```python
from build123d import *

# Parameters (mm, degrees)
F0_W     = 65
F0_H     = 83
F0_R     = 2.75
F1_DEPTH = 5
F2_SIZE  = 10


with BuildPart() as f1:
    # F0 (on Front) → F1 (new body)
    with BuildSketch(Plane.XZ):
        with Locations((32.5, 41.5)):
            Rectangle(F0_W, F0_H)
        with Locations((17, 14)):
            Circle(F0_R, mode=Mode.SUBTRACT)
        with Locations((47, 14)):
            Circle(F0_R, mode=Mode.SUBTRACT)
        with Locations((17, 74)):
            Circle(F0_R, mode=Mode.SUBTRACT)
        with Locations((47, 74)):
            Circle(F0_R, mode=Mode.SUBTRACT)
    extrude(amount=F1_DEPTH)

    # F2
    f2_edges = [f1.edges().sort_by_distance(p)[0] for p in [
        (65, -2.5, 0),
    ]]
    chamfer(f2_edges, length=F2_SIZE)


solid = f1.part
```
Verification items for the finished model (mm, model axes). Coordinates: 2 decimals unless noted, no trailing zeros. Loops run counter-clockwise (first coordinate to the right, second up) from the corner with the lowest first, then second, coordinate; pieces in that order, holes last. Notation, with made-up numbers: (-25, 33) -> (32, 33) arc R21 cw to (32, 55) -> close; hole circle Ø2 at (36, 14). An arc over 180 degrees is marked (long way). Answer in a Markdown table with one row per item. Add a question column.
1. Section check D-D, the plane x = 60. Enter the section's corners in (y, z), then the cut area to 3 significant figures.
2. Material ranges on probe 1 along Z at (x, y) = (17, -2.75); probe 2 along X at (y, z) = (-4.7, 15.5); probe 3 along X at (y, z) = (-0.7, 12), recorded low to high. Write a range as [from, to].
3. Section check A-A, the plane z = 14. Enter the section's corners in (x, y), then the cut area to 3 significant figures.
4. Section check C-C, the plane y = -2.8. Enter the section's corners in (x, z), then the cut area to 3 significant figures.
5. Draft check along Z on faces 1 (the face through (16.642, -2.465, 76.727)), 2 (the face through (60, -2, 5)), 3 (the face through (0, -2, 41)), 4 (the face through (14.973, -2.465, 15.859)). Enter one of: +Z half, -Z half, draft (parallel to the pull), parting line (faces both ways), or undercut.
6. Section check B-B, the plane x = 47. Enter the section's corners in (y, z).
Derived:
| question | item | result |
|---|---|---|
| 1 | outline | (-5, 5) -> (0, 5) -> (0, 83) -> (-5, 83) -> close |
| 1 | area | 390 mm² |
| 2 | probe 1 | z = [0, 11.25], [16.75, 71.25], [76.75, 83] |
| 2 | probe 2 | x = [0, 14.7], [19.3, 44.7], [49.3, 65] |
| 2 | probe 3 | x = [0, 15.11], [18.89, 45.11], [48.89, 65] |
| 3 | outline | (0, -5) -> (14.25, -5) -> (14.25, 0) -> (0, 0) -> close; (19.75, -5) -> (44.25, -5) -> (44.25, 0) -> (19.75, 0) -> close; (49.75, -5) -> (65, -5) -> (65, 0) -> (49.75, 0) -> close |
| 3 | area | 270 mm² |
| 4 | outline | (0, 0) -> (55, 0) -> (65, 10) -> (65, 83) -> (0, 83) -> close; hole circle Ø5.5 at (17, 14); hole circle Ø5.5 at (17, 74); hole circle Ø5.5 at (47, 14); hole circle Ø5.5 at (47, 74) |
| 4 | area | 5,250 mm² |
| 5 | face 1 | undercut |
| 5 | face 2 | -Z half |
| 5 | face 3 | draft |
| 5 | face 4 | undercut |
| 6 | outline | (-5, 0) -> (0, 0) -> (0, 11.25) -> (-5, 11.25) -> close; (-5, 16.75) -> (0, 16.75) -> (0, 71.25) -> (-5, 71.25) -> close; (-5, 76.75) -> (0, 76.75) -> (0, 83) -> (-5, 83) -> close |
